Can you work these out from the model? Positions are in its coordinate system, mm. A direction names the side the tool comes from. Give positions to 0.01 mm unless a question says otherwise; leave off trailing zeros. Order: outer loops, then holes, each group sorted by start corner. A loop starts at its lowest first (then second) coordinate and runs counter-clockwise, first axis right, second up. Notation, with made-up numbers: (-38.75, -21.5) - (15.25, -21.5) arc R21 cw to (15.25, 13.5) - close; hole circle Ø5 at (-26, 83). An arc over 180 degrees is marked (long way). Answer as a JSON object with one key per item and string values.
Autodesk Inventor part; units mm, degrees
ref_plane "YZ Plane" through (0, 0, 0) normal (1, 0, 0) x (0, 1, 0)
ref_plane "XZ Plane" through (0, 0, 0) normal (0, 1, 0) x (-1, 0, 0)
ref_plane "XY Plane" through (0, 0, 0) normal (0, 0, 1) x (1, 0, 0)
sketch "スケッチ1" plane through (0, 0, 0) normal (0, 1, 0) x (-1, 0, 0)
  line L0 (-4.45, 12) -> (4.45, 12)
  line L1 (4.45, 12) -> (4.45, -12)
  line L2 (4.45, -12) -> (-4.45, -12)
  line L3 (-4.45, -12) -> (-4.45, 12)
  point P0 (0, 0)
  dimension "d0" = 8.9
  dimension "d2" = 24
  dimension "d3" = 4.45
  dimension "d4" = 12
extrude "押し出し1" add sketch "スケッチ1" along normal blind 1.9
sketch "スケッチ4" plane through (0, 0, 0) normal (0, -1, 0) x (1, 0, 0)
  line L0 (4.45, 12) -> (-4.45, 12)
  line L1 (-4.45, -12) -> (4.45, -12)
  line L2 (4.45, -12) -> (4.45, 12)
  line L3 (-2.8, 12) -> (1.45, 12)
  line L4 (1.45, 12) -> (1.45, -6)
  line L5 (1.45, -6) -> (-2.8, -6)
  line L6 (-2.8, -6) -> (-2.8, 12)
  point P0 (0, 0)
  dimension "d39" = 6
  dimension "d40" = 4.25
  dimension "d41" = 3
extrude "押し出し3" cut sketch "スケッチ4" against normal blind 0.5
sketch "スケッチ3" plane through (0, 1.9, 0) normal (0, 1, 0) x (1, 0, 0)
  line L0 (-4.45, -12) -> (4.45, -12)
  line L1 (4.45, 12) -> (-4.45, 12)
  line L2 (-4.45, 12) -> (-4.45, -12)
  line L3 (-3.45, -12) -> (-0.45, -12)
  line L4 (-0.45, -12) -> (-0.45, 12)
  line L5 (-0.45, 12) -> (-3.45, 12)
  line L6 (-3.45, 12) -> (-3.45, -12)
  line L7 (1.05, 12) -> (2.55, 12)
  line L8 (2.55, 12) -> (2.55, -12)
  line L9 (2.55, -12) -> (1.05, -12)
  line L10 (1.05, -12) -> (1.05, 12)
  point P0 (0, 0)
  dimension "d35" = 1
  dimension "d36" = 3
  dimension "d37" = 1.5
  dimension "d38" = 1.5
extrude "押し出し4" cut sketch "スケッチ3" against normal blind 0.5 contours L6 L1 L4 L0 | L10 L1 L8 L0
sketch "スケッチ2" plane through (0, 1.9, 0) normal (0, 1, 0) x (1, 0, 0)
  line L0 (-4.45, -12) -> (4.45, -12)
  line L1 (4.45, 12) -> (-4.45, 12)
  line L2 (-4.45, 12) -> (-4.45, -12)
  line L3 (-4.45, -12) -> (-3.25, -12)
  line L4 (-3.25, -12) -> (-3.25, 6)
  line L5 (-3.25, 6) -> (-4.45, 6)
  line L6 (-4.45, 6) -> (-4.45, -12)
  line L7 (4.45, -12) -> (3.25, -12)
  line L8 (3.25, -12) -> (3.25, 6)
  line L9 (3.25, 6) -> (4.45, 6)
  line L10 (4.45, 6) -> (4.45, -12)
  line L11 (1.75, -12) -> (3.25, -10.5)
  line L12 (-2.35, -12) -> (-2.35, 6)
  line L13 (-2.35, 6) -> (-3.25, 6)
  line L14 (1.65, -12) -> (-2.35, -8)
  line L15 (-2.35, -7.1) -> (-2.15, -6.9)
  line L16 (-2.15, -6.9) -> (-2.35, -6.7)
  line L17 (-2.35, -5.8) -> (-0.35, -3.8)
  line L18 (-0.35, -3.8) -> (-2.35, -1.8)
  line L19 (-2.35, -0.9) -> (-2.15, -0.7)
  line L20 (-2.15, -0.7) -> (-2.35, -0.5)
  line L21 (-2.35, 0.4) -> (-0.35, 2.4)
  line L22 (-0.35, 2.4) -> (-3.25, 5.3)
  line L23 (1.65, -12) -> (1.75, -12)
  line L24 (2.55, -12) -> (2.55, 12)
  line L25 (2.55, 12) -> (4.45, 12)
  line L26 (4.45, 12) -> (4.45, -12)
  line L27 (4.45, -12) -> (2.55, -12)
  line L28 (-0.45, -12) -> (-0.45, 12)
  line L29 (-0.45, 12) -> (1.05, 12)
  line L30 (1.05, 12) -> (1.05, -12)
  line L31 (1.05, -12) -> (-0.45, -12)
  line L32 (-3.45, 12) -> (-3.45, -12)
  line L33 (-3.45, -12) -> (-4.45, -12)
  line L34 (-4.45, -12) -> (-4.45, 12)
  line L35 (-4.45, 12) -> (-3.45, 12)
  point P0 (0, 0)
  dimension "d7" = 6.5
  dimension "d9" = 1.2
  dimension "d10" = 6
  dimension "d11" = 6
  dimension "d12" = 1.5
  dimension "d13" = 1.5
  dimension "d20" = 5.6
  dimension "d22" = 4
  dimension "d23" = 4
  dimension "d24" = 0.2
  dimension "d25" = 0.9
  dimension "d26" = 0.9
  dimension "d27" = 2
  dimension "d28" = 0.2
  dimension "d29" = 0.9
  dimension "d30" = 2
  dimension "d31" = 0.9
  dimension "d32" = 135
extrude "押し出し5" cut sketch "スケッチ2" against normal blind 2 contours L32 L1 L28 L22 L12 L13 L5 | L4 L13 L12 L22 | L12 L15 L16 L17 L28 L14 | L1 L30 L14 L28 L17 L18 L21 L22 | L21 L28 L18 L12 L19 L20 | L1 L24 L11 L0 L14 L30 | L1 L26 L9 L8 L11 L24 keep common part
fillet "フィレット1" radius 0.2 6 edges at (-2.15, 0.95, 0.7) (-2.15, 0.95, 6.9) (-2.35, 0.95, 0.5) (-2.35, 0.95, 0.9) (-2.35, 0.95, 6.7) (-2.35, 0.95, 7.1)
properties part number "key"
Q1. We'd pull the mould along Z, two halves only. Please class faces 4 (the face through (2.49, 0.96, 11.26)), 5 (the face through (-1.78, 0.96, -3.83)), 6 (the face through (0, 0.5, 3)): released by +Z, released by -Z, zero draft, split by the parting line, or undercut.
Recorded:
{"face 4": "released by +Z", "face 5": "undercut", "face 6": "zero draft"}
Q2. If we section it at B-B, the plane z = 7.5: Please give me the cut outline in (x, y), then the cut area to 3 significant figures.
Recorded:
{"outline": "(-2.35, 0.5) - (1.45, 0.5) - (1.45, 0) - (3.25, 0) - (3.25, 1.9) - (2.55, 1.9) - (2.55, 1.4) - (1.05, 1.4) - (1.05, 1.9) - (-0.45, 1.9) - (-0.45, 1.4) - (-2.35, 1.4) - close", "area": "7.04 mm^2"}
Q3. I need wall thicknesses on L1, parallel to X at y = 1.7, z = 4; L2, parallel to X at y = 0.1, z = 2.5; L3, parallel to Z at x = -0.25, y = 0.3. Which ranges of each line are inside material? Lowest first, please.
Recorded:
{"L1": "x = -0.45 to 1.05, 2.55 to 3.25", "L2": "x = 1.45 to 3.25", "L3": "z = -12 to -6"}
Q4. Which directions (+Z, -Z, +X, -X, +Y, -Y) give clear straight access to the entire face, cutting with the end or side of a thin tool? Please do faces 1 (the face through (-2.35, 1, 6)), 2 (the face through (-1.34, 1.05, 2.81)), 3 (the face through (-2, 1.4, -8)).
Recorded:
{"face 1": "+Z, -X, +Y, -Y", "face 2": "-X, +Y, -Y", "face 3": "+Z, -Z, -X, +Y"}
Q5. I'm going to push flat-ended pins straight in: pin 1 Ø0.9 at (y, z) = (1, 1.5) entering from -X; pin 2 Ø1 at (x, y) = (3.5, 0.5) entering from +Z; pin 3 Ø1.5 at (x, z) = (-1.5, 5.5) entering from +Y. Where does each tip first touch, or does it pass through?
Recorded:
{"pin 1": "stops at x = -2.35", "pin 2": "stops at z = 10.75", "pin 3": "stops at y = 1.4"}
Q6. If we section it at A-A, the plane x = -2: Please give me the cut outline in (y, z).
Recorded:
{"outline": "(0, -12) - (1.4, -12) - (1.4, -4.05) - (0.5, -4.05) - (0.5, -6) - (0, -6) - close; (0.5, -0.75) - (1.4, -0.75) - (1.4, 2.15) - (0.5, 2.15) - close; (0.5, 5.45) - (1.4, 5.45) - (1.4, 8.35) - (0.5, 8.35) - close"}
Q7. If we section it at D-D, the plane x = 0.5: Please give me the cut outline in (y, z), then the cut area to 3 significant figures.
Recorded:
{"outline": "(0, -12) - (1.9, -12) - (1.9, 10.85) - (0.5, 10.85) - (0.5, -6) - (0, -6) - close", "area": "35.0 mm^2"}
